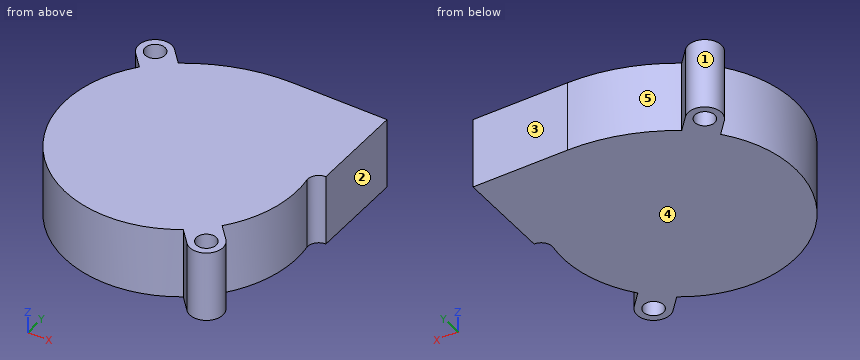
```python
from build123d import *

# Parameters (mm, degrees)
SKETCH1_R           = 2.1
BOSS_EXTRUDE1_DEPTH = 15


with BuildPart() as part:
    # Sketch1 → Boss-Extrude1 (new body)
    with BuildSketch(Plane.XY):
        with BuildLine():
            Line((-21.595375227, 18.651803366), (-18.864158731, 15.633090397))
            ThreePointArc((-18.864158731, 15.633090397), (-18.167626589, -16.437376437), (13.673408277, -20.329483665))
            Line((13.673408277, -20.329483665), (16.404624773, -23.348196634))
            ThreePointArc((16.404624773, -23.348196634), (21.348196634, -23.595375227), (21.595375227, -18.651803366))
            Line((21.595375227, -18.651803366), (18.864158731, -15.633090397))
            ThreePointArc((18.864158731, -15.633090397), (23.626039946, -6.485386377), (24.201713513, 3.811438449))
            ThreePointArc((24.201713513, 3.811438449), (24.731491872, 5.685176303), (26.5, 6.5))
            Line((26.5, 6.5), (26.5, 26.5))
            Line((26.5, 26.5), (6.557177663, 26.5))
            ThreePointArc((6.557177663, 26.5), (-4.018169605, 24.923070714), (-13.673408277, 20.329483665))
            Line((-13.673408277, 20.329483665), (-16.404624773, 23.348196634))
            ThreePointArc((-16.404624773, 23.348196634), (-21.348196634, 23.595375227), (-21.595375227, 18.651803366))
        make_face()
        with Locations((-19, 21)):
            Circle(SKETCH1_R, mode=Mode.SUBTRACT)
        with Locations((19, -21)):
            Circle(SKETCH1_R, mode=Mode.SUBTRACT)
    extrude(amount=BOSS_EXTRUDE1_DEPTH)


solid = part.part
```
Design review of the part built by this model. Coordinates are the model's own, in mm. Face numbers are marked on the shaded views. A direction names the side the tool comes from. Round coordinates to 2 decimals unless told otherwise and drop trailing zeros. Order: outer loops, then holes, each group sorted by start corner. A loop starts at its lowest first (then second) coordinate and runs counter-clockwise, first axis right, second up. Notation, with made-up numbers: (-32.5, 52) - (-5.5, 52) arc R26 cw to (-5.5, 70) - close; hole circle Ø1 at (36.5, 51.25). An arc over 180 degrees is marked (long way). Return JSON: item names as keys, results as strings.
Q1. Consider section B-B on z = 4.75. Write out the cut boundary in (x, y), plus the area to 3 significant figures.
Computed values:
{"outline": "(-21.6, 18.65) - (-18.86, 15.63) arc R24.5 ccw to (13.67, -20.33) - (16.4, -23.35) arc R3.5 ccw to (21.6, -18.65) - (18.86, -15.63) arc R24.5 ccw to (24.2, 3.81) arc R2.33 cw to (26.5, 6.5) - (26.5, 26.5) - (6.56, 26.5) arc R36.25 ccw to (-13.67, 20.33) - (-16.4, 23.35) arc R3.5 ccw to start; hole circle Ø4.2 at (-19, 21); hole circle Ø4.2 at (19, -21)", "area": "2,170 mm2"}
Q2. Consider section A-A on y = -21. Write out the cut boundary in (x, z).
Computed values:
{"outline": "(-12.62, 0) - (12.62, 0) - (12.62, 15) - (-12.62, 15) - close; (14.28, 0) - (16.9, 0) - (16.9, 15) - (14.28, 15) - close; (21.1, 0) - (22.5, 0) - (22.5, 15) - (21.1, 15) - close"}
Q3. Machinability: for the marked faces 4 and 5, which of the approach directions +Z, -Z, +X, -X, +Y, -Y give a long, thin tool a straight path to every point of the face, cutting with its end or side? Answer none if there is none.
Computed values:
{"face 4": "-Z, +X, -X, +Y, -Y", "face 5": "+Z, -Z, +Y"}
Q4. The part is to be moulded in two halves that separate along Y. For the marked faces 1, 2 and 3, say which applies: pulls with the +Y half, pulls with the -Y half, needs draft (parallel to the pull), parting line crosses it, or undercut.
Computed values:
{"face 1": "undercut", "face 2": "needs draft", "face 3": "pulls with the +Y half"}
Q5. Consider section D-D on y = 21. Write out the cut boundary in (x, z).
Computed values:
{"outline": "(-22.5, 0) - (-21.1, 0) - (-21.1, 15) - (-22.5, 15) - close; (-16.9, 0) - (-14.28, 0) - (-14.28, 15) - (-16.9, 15) - close; (-12.64, 0) - (26.5, 0) - (26.5, 15) - (-12.64, 15) - close"}
Q6. For pin 1 Ø3 at (x, z) = (-13.5, 7.5) entering from +Y; pin 2 Ø8 at (x, y) = (-12.5, -10) entering from -Z; pin 3 Ø4 at (x, y) = (-19, 21) entering from +Z; pin 4 Ø1 at (x, z) = (-13.5, 5) entering from -Y, all flat-tipped, find the tip position at first contact; note any pin that passes through.
Computed values:
{"pin 1": "stops at y = 21.8", "pin 2": "stops at z = 0", "pin 3": "passes through", "pin 4": "stops at y = -20.77"}
Q7. Wall thickness on L1, parallel to Y at x = 19, z = 12.25; L2, parallel to Y at x = -19, z = 5; L3, parallel to X at y = 18.5, z = 13.5: over which ranges is each line inside the solid? List them lowest first. Write a range as [from, to].
Computed values:
{"L1": "y = [-24.5, -23.1], [-18.9, -15.78], [-15.47, 26.5]", "L2": "y = [-15.47, 15.47], [15.78, 18.9], [23.1, 24.5]", "L3": "x = [-21.46, 26.5]"}
Q8. Consider section C-C on y = 0. Write out the cut boundary in (x, z), plus the area to 3 significant figures.
Computed values:
{"outline": "(-24.5, 0) - (24.5, 0) - (24.5, 15) - (-24.5, 15) - close", "area": "735 mm2"}
